from build123d import *

# Parameters (mm, degrees)
SKETCH_1_R          = 2.5
EXTRUDE_1_DEPTH     = 24
CUT_EXTRUDE_1_DEPTH = 11
SKETCH_3_R          = 2.5
EXTRUDE_2_DEPTH     = 2


with BuildPart() as part:
    # Эскиз1 → Бобышка-Вытянуть1 (new body)
    with BuildSketch(Plane(origin=(0, 0, 0), x_dir=(0, 0, -1), z_dir=(1, 0, 0))):
        with BuildLine():
            Line((-25, 9), (25, 9))
            ThreePointArc((25, 9), (26.414213562, 8.414213562), (27, 7))
            Line((27, 7), (27, -7))
            ThreePointArc((27, -7), (26.414213562, -8.414213562), (25, -9))
            Line((25, -9), (-25, -9))
            ThreePointArc((-25, -9), (-26.414213562, -8.414213562), (-27, -7))
            Line((-27, -7), (-27, 7))
            ThreePointArc((-27, 7), (-26.414213562, 8.414213562), (-25, 9))
        make_face()
        with Locations((-13.5, 0)):
            Circle(SKETCH_1_R, mode=Mode.SUBTRACT)
        with Locations((13.5, 0)):
            Circle(SKETCH_1_R, mode=Mode.SUBTRACT)
    extrude(amount=EXTRUDE_1_DEPTH)

    # Эскиз2 → Вырез-Вытянуть1 (cut)
    with BuildSketch(Plane(origin=(24, 0, 0), x_dir=(0, 0, -1), z_dir=(1, 0, 0))):
        with BuildLine():
            Line((-24.420860707, 9), (-24.420860707, 4.973409436))
            ThreePointArc((-24.420860707, 4.973409436), (-25.5, 0), (-24.420860707, -4.973409436))
            Line((-24.420860707, -4.973409436), (-24.420860707, -9))
            Line((-24.420860707, -9), (-2.579139293, -9))
            Line((-2.579139293, -9), (-2.579139293, -4.973409436))
            ThreePointArc((-2.579139293, -4.973409436), (-1.5, 0), (-2.579139293, 4.973409436))
            Line((-2.579139293, 4.973409436), (-2.579139293, 9))
            Line((-2.579139293, 9), (-24.420860707, 9))
        make_face()
        with BuildLine():
            Line((24.420860707, -4.973409436), (24.420860707, -9))
            Line((24.420860707, -9), (2.579139293, -9))
            Line((2.579139293, -9), (2.579139293, -4.973409436))
            ThreePointArc((2.579139293, -4.973409436), (1.5, 0), (2.579139293, 4.973409436))
            Line((2.579139293, 4.973409436), (2.579139293, 9))
            Line((2.579139293, 9), (24.420860707, 9))
            Line((24.420860707, 9), (24.420860707, 4.973409436))
            ThreePointArc((24.420860707, 4.973409436), (25.5, 0), (24.420860707, -4.973409436))
        make_face()
    extrude(amount=-CUT_EXTRUDE_1_DEPTH, mode=Mode.SUBTRACT)

    # Эскиз3 → Бобышка-Вытянуть2 (add)
    with BuildSketch(Plane(origin=(24, 0, 0), x_dir=(0, 0, -1), z_dir=(1, 0, 0))):
        with BuildLine():
            Line((-25, 9), (25, 9))
            ThreePointArc((25, 9), (26.414213562, 8.414213562), (27, 7))
            Line((27, 7), (27, -7))
            ThreePointArc((27, -7), (26.414213562, -8.414213562), (25, -9))
            Line((25, -9), (-25, -9))
            ThreePointArc((-25, -9), (-26.414213562, -8.414213562), (-27, -7))
            Line((-27, -7), (-27, 7))
            ThreePointArc((-27, 7), (-26.414213562, 8.414213562), (-25, 9))
        make_face()
        with Locations((-13.5, 0)):
            Circle(SKETCH_3_R, mode=Mode.SUBTRACT)
        with Locations((13.5, 0)):
            Circle(SKETCH_3_R, mode=Mode.SUBTRACT)
    extrude(amount=EXTRUDE_2_DEPTH)


solid = part.part
Check sheet for the modelled part. Datum: model origin and axes. Units: mm. A direction names the side the tool comes from. Round coordinates to 2 decimals unless told otherwise and drop trailing zeros. Write each loop counter-clockwise with the first axis right and the second up, starting at its lowest first coordinate (ties: lowest second). Pieces come first, ordered by that corner, then holes. Notation, with made-up numbers: (46.25, -3) -> (90.25, -3) arc R25 cw to (90.25, 33) -> close; hole circle Ø2 at (50.5, -20.75). An arc over 180 degrees is marked (long way). Answer as CSV lines item,"result". Start each with the question number.
1) Tool access check on faces 1 (the cylindrical face through (12.82, 8.43, -26.4)), 2 (the flat face through (19, 7, -2.579)). Record the directions out of +Z, -Z, +X, -X, +Y, -Y that give a thin tool (end or side, any length) a straight path to the whole face; none if there is none.
2) Section check D-D on x = 9.5. Enter the section's corners in (y, z).
3) Section check A-A on x = 21. Enter the section's corners in (y, z).
4) Material ranges on line 1 (Z direction, x = 5.5, y = 0); line 2 (Z direction, x = 21, y = 6.75); line 3 (X direction, y = -6.25, z = 8.5), recorded low to high. Write a range as from..to.
5) Release check for a two-part mould opening along Y. For faces 3 (the cylindrical face through (18.6, 0.1, -25.5)), 4 (the cylindrical face through (12.82, -8.43, 26.4)), 5 (the flat face through (19, 7, 2.579)), 6 (the cylindrical face through (18.6, -0.1, -1.5)) record: pulls with the +Y half, pulls with the -Y half, needs draft (parallel to the pull), parting line crosses it, or undercut.
6) Section check B-B on z = 17. Enter the section's corners in (x, y), and give its area (3 significant figures).
7) Section check C-C on y = 0. Enter the section's corners in (x, z), and give its area (3 significant figures).
8) Go/stop test with flat-tipped pins: P1, Ø6.5, axis at y = 0, z = -13.5, coming from the -X side; P2, Ø4.5, axis at y = 0, z = 13.5, coming from the -X side. Record where each tip stops, or that it passes through.
Found:
1,face 1,"-Z, +X, -X, +Y"
1,face 2,"+Y, -Y"
2,outline,"(-9, -25) arc R2 ccw to (-7, -27) -> (7, -27) arc R2 ccw to (9, -25) -> (9, 25) arc R2 ccw to (7, 27) -> (-7, 27) arc R2 ccw to (-9, 25) -> close; hole circle Ø5 at (0, -13.5); hole circle Ø5 at (0, 13.5)"
3,outline,"(-9, -25) arc R2 ccw to (-7, -27) -> (7, -27) arc R2 ccw to (9, -25) -> (9, -24.42) -> (4.97, -24.42) arc R12 cw to (-4.97, -24.42) -> (-9, -24.42) -> close; (-9, -2.58) -> (-4.97, -2.58) arc R12 cw to (4.97, -2.58) -> (9, -2.58) -> (9, 2.58) -> (4.97, 2.58) arc R12 cw to (-4.97, 2.58) -> (-9, 2.58) -> close; (-9, 24.42) -> (-4.97, 24.42) arc R12 cw to (4.97, 24.42) -> (9, 24.42) -> (9, 25) arc R2 ccw to (7, 27) -> (-7, 27) arc R2 ccw to (-9, 25) -> close"
4,line 1,"z = -27..-16, -11..11, 16..27"
4,line 2,"z = -27..-24.42, -2.58..2.58, 24.42..27"
4,line 3,"x = 0..13, 24..26"
5,face 3,"undercut"
5,face 4,"pulls with the -Y half"
5,face 5,"needs draft"
5,face 6,"undercut"
6,outline,"(0, -9) -> (13, -9) -> (13, 9) -> (0, 9) -> close; (24, -9) -> (26, -9) -> (26, 9) -> (24, 9) -> close"
6,area,"270 mm^2"
7,outline,"(0, -27) -> (26, -27) -> (26, -16) -> (24, -16) -> (24, -25.5) -> (13, -25.5) -> (13, -16) -> (0, -16) -> close; (0, -11) -> (13, -11) -> (13, -1.5) -> (24, -1.5) -> (24, -11) -> (26, -11) -> (26, 11) -> (24, 11) -> (24, 1.5) -> (13, 1.5) -> (13, 11) -> (0, 11) -> close; (0, 16) -> (13, 16) -> (13, 25.5) -> (24, 25.5) -> (24, 16) -> (26, 16) -> (26, 27) -> (0, 27) -> close"
7,area,"726 mm^2"
8,P1,"stops at x = 0"
8,P2,"passes through"
